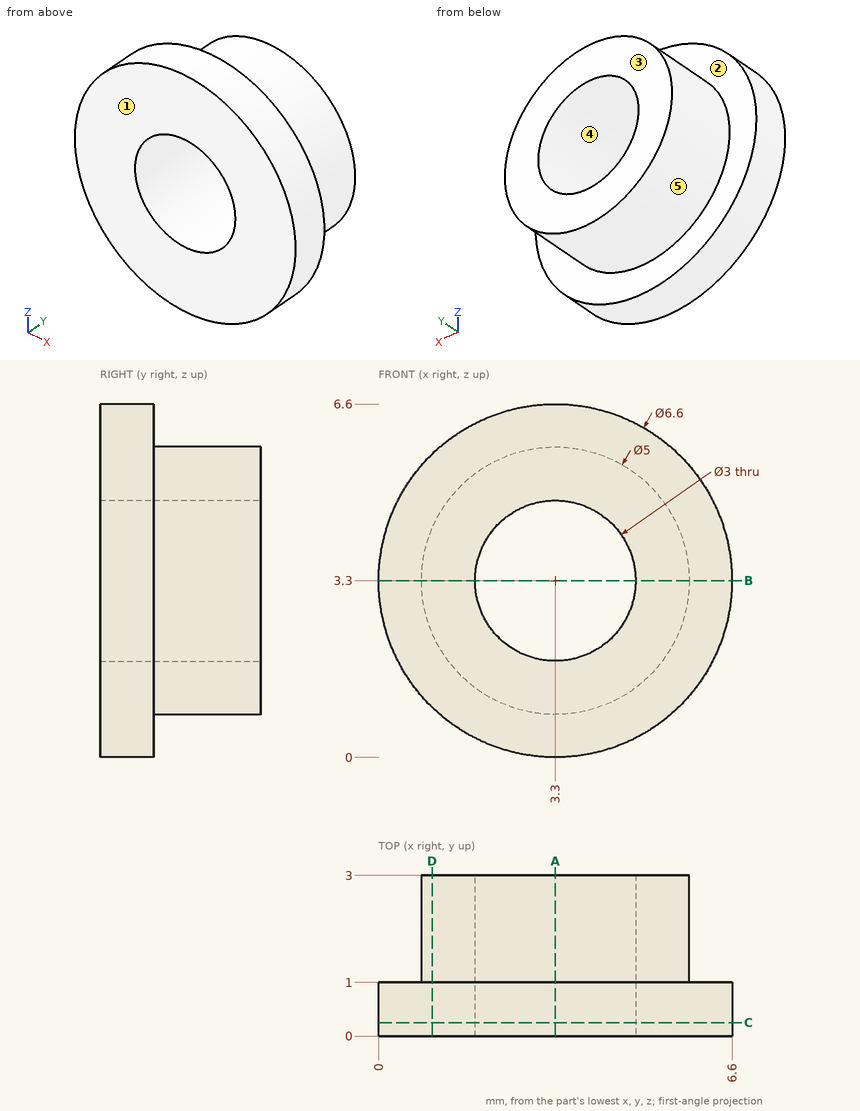
Print and shaded views of the part. All mm, measured from the part's lowest x, y and z. A direction names the side the tool comes from. Round coordinates to 2 decimals unless told otherwise and drop trailing zeros. Write each loop counter-clockwise with the first axis right and the second up, starting at its lowest first coordinate (ties: lowest second). Pieces come first, ordered by that corner, then holes.
(1) Slice it at B-B, the plane z = 3.3. Write the cut outline in (x, y).
(2) Slice it at C-C, the plane y = 0.25. Write the cut outline in (x, z).
(3) Slice it at A-A, the plane x = 3.3. Write the cut outline in (y, z).
(4) Slice it at D-D, the plane x = 1. Write the cut outline in (y, z), and give its area (3 significant figures).
(5) Probe line 1 along X through (y, z) = (2.35, 3.3); line 2 along Y through (x, z) = (4.75, 1). List the from-to ranges inside material, lowest first.
(6) Mould opens along X. For the marked faces 3, 4 and 5 say: pulls with the +X half, pulls with the -X half, needs draft (parallel to the pull), parting line crosses it, or undercut.
(7) 3-axis set-ups, long thin cutter, end or side, ignore diameter. For the marked faces 1 and 2: which of +Z, -Z, +X, -X, +Y, -Y reach the whole face in a straight line?
(8) Drop flat-ended pins along their axis: P1, Ø1.5, axis at y = 2, z = 4, coming from the +X side; P2, Ø1, axis at y = 1, z = 2, coming from the -X side; P3, Ø1.5, axis at x = 4.5, z = 4, coming from the +Y side; P4, Ø2.5, axis at x = 3.3, z = 3.3, coming from the -Y side. Give the stop position or say it passes through.
From the geometry:
1. outline: (0, 0) - (1.8, 0) - (1.8, 3) - (0.8, 3) - (0.8, 1) - (0, 1) - close; (4.8, 0) - (6.6, 0) - (6.6, 1) - (5.8, 1) - (5.8, 3) - (4.8, 3) - close
2. outline: circle Ø6.6 at (3.3, 3.3); hole circle Ø3 at (3.3, 3.3)
3. outline: (0, 0) - (1, 0) - (1, 0.8) - (3, 0.8) - (3, 1.8) - (0, 1.8) - close; (0, 4.8) - (3, 4.8) - (3, 5.8) - (1, 5.8) - (1, 6.6) - (0, 6.6) - close
4. outline: (0, 0.93) - (1, 0.93) - (1, 2.32) - (3, 2.32) - (3, 4.28) - (1, 4.28) - (1, 5.67) - (0, 5.67) - close
4. area: 8.65 mm2
5. line 1: x = 0.8 to 1.8, 4.8 to 5.8
5. line 2: y = 0 to 1
6. face 3: needs draft
6. face 4: undercut
6. face 5: parting line crosses it
7. face 1: +Z, -Z, +X, -X, -Y
7. face 2: +Y
8. P1: stops at x = 5.8
8. P2: stops at x = 0.1
8. P3: stops at y = 3
8. P4: passes through
